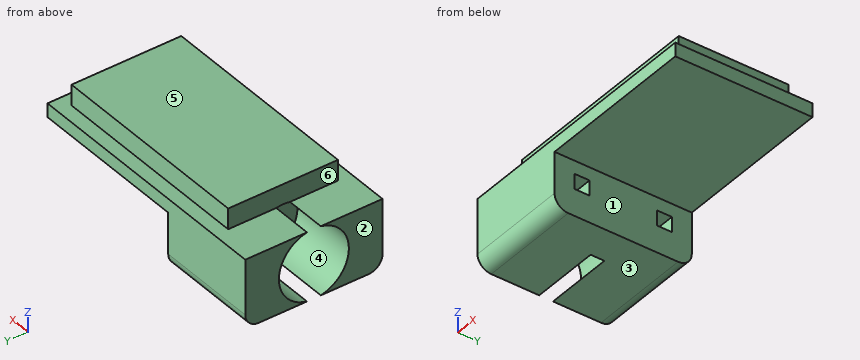
```python
from build123d import *

# Parameters (mm, degrees)
SKETCH1_W           = 20
SKETCH1_H           = 10
BOSS_EXTRUDE1_DEPTH = 38.5
SKETCH5_W           = 16
SKETCH5_H           = 30.5
BOSS_EXTRUDE2_DEPTH = 8
SKETCH2_R           = 5.1
CUT_EXTRUDE3_DEPTH  = 10
FILLET1_R           = 2
SKETCH6_W           = 23.5
SKETCH6_H           = 20
CUT_EXTRUDE4_DEPTH  = 8
SKETCH7_W           = 2.2
SKETCH7_H           = 2.2
CUT_EXTRUDE5_DEPTH  = 3


with BuildPart() as part:
    # Sketch1 → Boss-Extrude1 (new body)
    with BuildSketch(Plane.YZ):
        Rectangle(SKETCH1_W, SKETCH1_H)
    extrude(amount=BOSS_EXTRUDE1_DEPTH)

    # Sketch5 → Boss-Extrude2 (add)
    with BuildSketch(Plane(origin=(0, 0, 0), x_dir=(0, 1, 0), z_dir=(0, 0, 1))):
        with Locations((0, -21.25)):
            Rectangle(SKETCH5_W, SKETCH5_H)
    extrude(amount=BOSS_EXTRUDE2_DEPTH)

    # Sketch2 → Cut-Extrude3 (cut)
    with BuildSketch(Plane.YZ):
        Circle(SKETCH2_R)
    extrude(amount=CUT_EXTRUDE3_DEPTH, mode=Mode.SUBTRACT)

    # Fillet1
    fillet1_edges = [part.edges().sort_by_distance(p)[0] for p in [
        (19.25, 10, -5),
        (19.25, -10, -5),
    ]]
    fillet(fillet1_edges, radius=FILLET1_R)

    # Sketch6 → Cut-Extrude4 (cut)
    with BuildSketch(Plane(origin=(0, 0, -5), x_dir=(1, 0, 0), z_dir=(0, 0, -1))):
        with Locations((26.75, 0)):
            Rectangle(SKETCH6_W, SKETCH6_H)
    extrude(amount=-CUT_EXTRUDE4_DEPTH, mode=Mode.SUBTRACT)

    # Sketch7 → Cut-Extrude5 (cut)
    with BuildSketch(Plane.YZ.offset(15)):
        with Locations((6, 0)):
            Rectangle(SKETCH7_W, SKETCH7_H)
        with Locations((-6, 0)):
            Rectangle(SKETCH7_W, SKETCH7_H)
    extrude(amount=-CUT_EXTRUDE5_DEPTH, mode=Mode.SUBTRACT)


solid = part.part
```
Input: part model. Units: mm. Frame: model coordinates. Face numbers are marked on the shaded views. A direction names the side the tool comes from. Coordinates: 2 decimals unless noted, no trailing zeros. Write each loop counter-clockwise with the first axis right and the second up, starting at its lowest first coordinate (ties: lowest second). Pieces come first, ordered by that corner, then holes.
1) Pin query (flat end, axial travel): pin 1 Ø1.5 at (y, z) = (2.5, 7) entering from +X; pin 2 Ø3.5 at (y, z) = (-3, 6) entering from -X; pin 3 Ø4 at (y, z) = (-4.5, 0.5) entering from +X; pin 4 Ø2.5 at (x, z) = (21.5, 7) entering from +Y. Return the tip coordinate at first contact, or that it passes through.
2) Set-up query: the marked faces 1 and 2. Return all of +Z, -Z, +X, -X, +Y, -Y with unobstructed straight access to the full face (end or side cutting, diameter ignored); none if empty.
3) Mould query, pull axis Z, two halves, no side actions, for the marked faces 3, 4, 5 and 6. Classes: pulls with the +Z half, pulls with the -Z half, needs draft (parallel to the pull), parting line crosses it, or undercut.
4) Section D-D on z = 1.75. Output: boundary loops of the cut face in (x, y).
5) Section B-B on y = 0. Output: boundary loops of the cut face in (x, z).
6) Section A-A on z = 0. Output: boundary loops of the cut face in (x, y), and give its area (3 significant figures).
7) Section C-C on x = 22. Output: boundary loops of the cut face in (y, z).
8) Material intervals for line 1 along Y through (x, z) = (6, 0); line 2 along X through (y, z) = (-0.5, 4.25); line 3 along X through (y, z) = (8.5, 1.5), sorted ascending.
Check result:
1. pin 1: stops at x = 36.5
1. pin 2: stops at x = 0
1. pin 3: stops at x = 15
1. pin 4: stops at y = 8
2. face 1: -Z, +X, +Y, -Y
2. face 2: +Z, -Z, -X, +Y, -Y
3. face 3: pulls with the -Z half
3. face 4: undercut
3. face 5: pulls with the +Z half
3. face 6: needs draft
4. outline: (0, -10) - (15, -10) - (15, 10) - (0, 10) - (0, 4.79) - (10, 4.79) - (10, -4.79) - (0, -4.79) - close
5. outline: (6, 5.1) - (10, 5.1) - (10, -5) - (15, -5) - (15, 3) - (38.5, 3) - (38.5, 5) - (36.5, 5) - (36.5, 8) - (6, 8) - close
6. outline: (0, -10) - (15, -10) - (15, -7.1) - (12, -7.1) - (12, -4.9) - (15, -4.9) - (15, 4.9) - (12, 4.9) - (12, 7.1) - (15, 7.1) - (15, 10) - (0, 10) - (0, 5.1) - (10, 5.1) - (10, -5.1) - (0, -5.1) - close
6. area: 185 mm2
7. outline: (-10, 3) - (10, 3) - (10, 5) - (8, 5) - (8, 8) - (-8, 8) - (-8, 5) - (-10, 5) - close
8. line 1: y = -10 to -5.1, 5.1 to 10
8. line 2: x = 10 to 38.5
8. line 3: x = 0 to 15
